Design review of the part shown in the three views and the two pictorial views. Dimensions are in mm from the part's minimum x, y and z. Round coordinates to 2 decimals unless told otherwise and drop trailing zeros. Loops run counter-clockwise (first coordinate to the right, second up) from the corner with the lowest first, then second, coordinate; pieces in that order, holes last. Notation, with made-up numbers: (54.5, 45) - (69.5, 45) arc R33 cw to (69.5, 82) - close; hole circle Ø9 at (37.25, -12). An arc over 180 degrees is marked (long way). Return JSON: item names as keys, results as strings. Group by question number.
(1) We need section A-A, the plane x = 455. Write out the cut boundary in (y, z).
(2) Wall thickness on L1, parallel to X at y = 9, z = 166 (1 decimal); L2, parallel to Z at x = 364, y = 3.5; L3, parallel to X at y = 16.5, z = 198.5 (1 decimal): over which ranges is each line inside the solid? List them lowest first. Write a range as [from, to].
(3) Clearance check with flat-ended pins moving along their axes: pin 1 (1.5 mm diameter, centred on y = 14.5, z = 612, fed in from -X); pin 2 (9.5 mm diameter, centred on x = 390.5, y = 10.5, fed in from +Z); pin 3 (9.5 mm diameter, centred on y = 14, z = 296, fed in from -X). State where each tip first meets the part, or that it passes through.
(4) We need section D-D, the plane z = 306. Write out the cut boundary in (x, y).
(5) We need section C-C, the plane y = 10.5. Write out the cut boundary in (x, z), and give its area (3 significant figures).
(6) We need section B-B, the plane x = 354. Write out the cut boundary in (y, z).
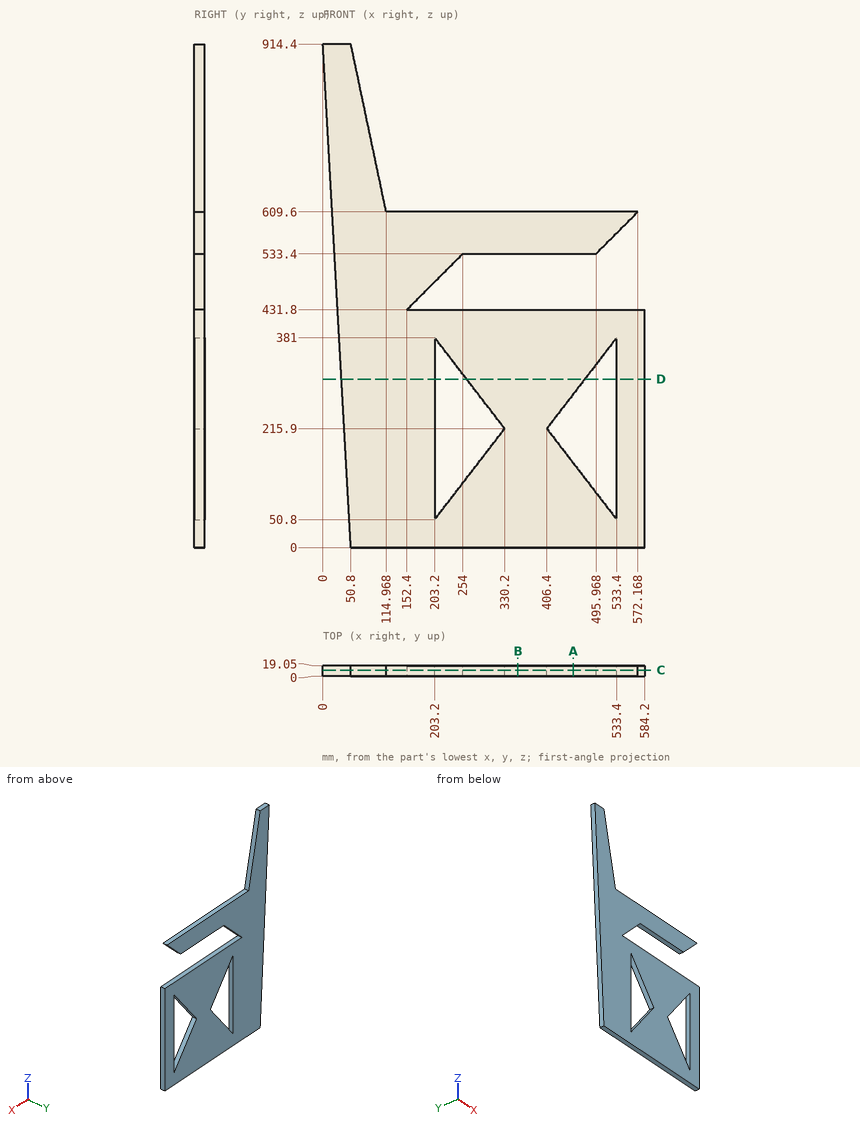
Solutions:
{
 "1": {"outline": "(0, 0) - (19.05, 0) - (19.05, 152.72) - (0, 152.72) - close; (0, 279.08) - (19.05, 279.08) - (19.05, 431.8) - (0, 431.8) - close; (0, 533.4) - (19.05, 533.4) - (19.05, 609.6) - (0, 609.6) - close"},
 "2": {"L1": "[41.6, 203.2], [291.8, 444.8], [533.4, 584.2]", "L2": "[0, 431.8], [533.4, 609.6]", "L3": "[39.8, 203.2], [316.8, 419.8], [533.4, 584.2]"},
 "3": {"pin 1": "x = 16.76", "pin 2": "z = 609.6", "pin 3": "x = 34.09"},
 "4": {"outline": "(33.8, 0) - (203.2, 0) - (203.2, 19.05) - (33.8, 19.05) - close; (260.89, 0) - (475.71, 0) - (475.71, 19.05) - (260.89, 19.05) - close; (533.4, 0) - (584.2, 0) - (584.2, 19.05) - (533.4, 19.05) - close"},
 "5": {"outline": "(0, 914.4) - (50.8, 0) - (584.2, 0) - (584.2, 431.8) - (152.4, 431.8) - (254, 533.4) - (495.97, 533.4) - (572.17, 609.6) - (114.97, 609.6) - (50.8, 914.4) - close; hole (203.2, 50.8) - (330.2, 215.9) - (203.2, 381) - close; hole (406.4, 215.9) - (533.4, 50.8) - (533.4, 381) - close", "area": "274,000 mm^2"},
 "6": {"outline": "(0, 0) - (19.05, 0) - (19.05, 431.8) - (0, 431.8) - close; (0, 533.4) - (19.05, 533.4) - (19.05, 609.6) - (0, 609.6) - close"}
}
